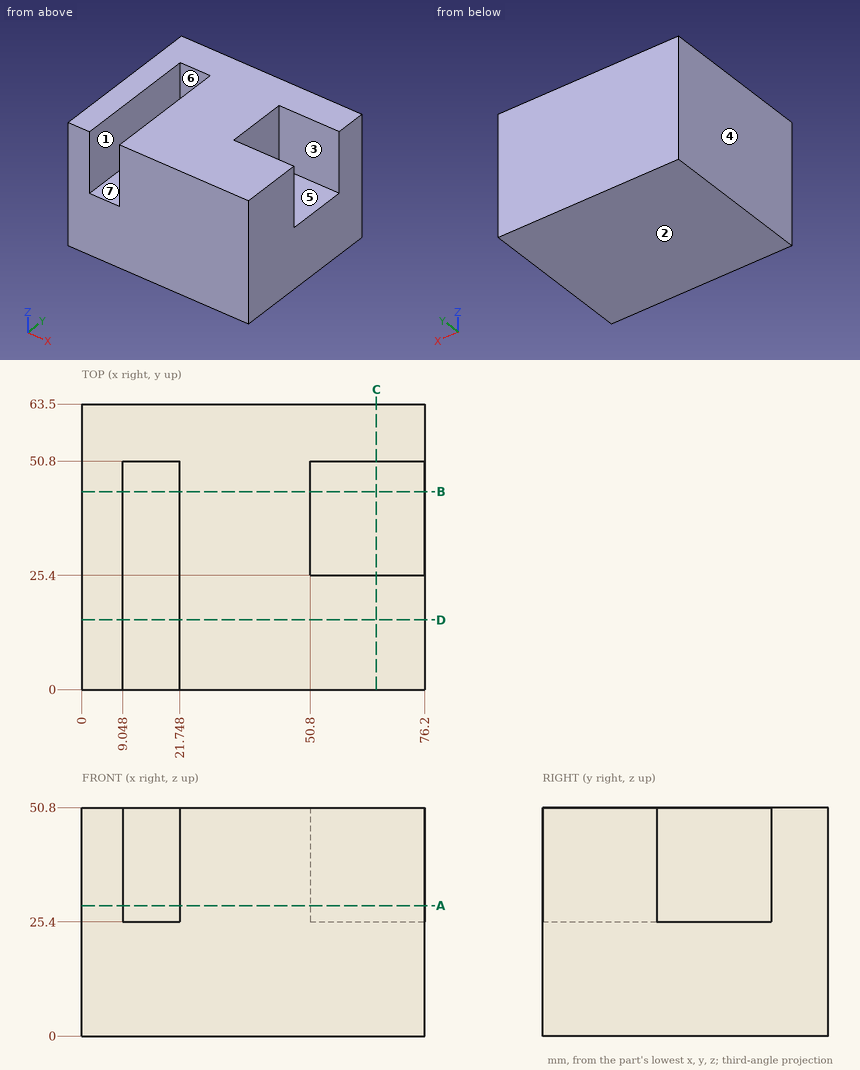
Geometry: see drawing. Coordinates: mm, zero at the bounding-box minimum. A direction names the side the tool comes from. Coordinates: 2 decimals unless noted, no trailing zeros. Order: outer loops, then holes, each group sorted by start corner. A loop starts at its lowest first (then second) coordinate and runs counter-clockwise, first axis right, second up. Notation, with made-up numbers: M 59.5,69.5 L 97.5,69.5 A17 ccw 97.5,84.5 Z; hole C -10.75,4.5 d3. An arc over 180 degrees is marked long. Answer in a Markdown table with one row per item. Add a question column.
Q1. Line query: L1, parallel to X at y = 44, z = 27; L2, parallel to X at y = 16, z = 49; L3, parallel to Y at x = 54.5, z = 43. Output: solid intervals per line, ascending.
Q2. Section query D-D on y = 15.5. Return the cut outline in (x, z), and give its area (3 significant figures).
Q3. Section query C-C on x = 65.5. Return the cut outline in (y, z).
Q4. Section query B-B on y = 44. Return the cut outline in (x, z).
Q5. Contact query for flat-ended pins moving along their axis: P1, Ø5, axis at x = 16, y = 11.5, coming from the +Z side; P2, Ø12, axis at y = 35, z = 44, coming from the +X side. Output: stop coordinate, or through.
Q6. Reachability of the marked faces 1, 2 and 3 from +Z, -Z, +X, -X, +Y, -Y: full face, straight path, thin tool, end or side. Return the list, or none.
Q7. Section query A-A on z = 29. Return the cut outline in (x, y).
Q8. Mould query, pull axis X, two halves, no side actions, for the marked faces 4, 5, 6 and 7. Classes: released by +X, released by -X, zero draft, split by the parting line, or undercut.
Completed:
| question | item | result |
|---|---|---|
| 1 | L1 | x = 0 to 9.05, 21.75 to 50.8 |
| 1 | L2 | x = 0 to 9.05, 21.75 to 76.2 |
| 1 | L3 | y = 0 to 25.4, 50.8 to 63.5 |
| 2 | outline | M 0,0 L 76.2,0 L 76.2,50.8 L 21.75,50.8 L 21.75,25.4 L 9.05,25.4 L 9.05,50.8 L 0,50.8 Z |
| 2 | area | 3,550 mm2 |
| 3 | outline | M 0,0 L 63.5,0 L 63.5,50.8 L 50.8,50.8 L 50.8,25.4 L 25.4,25.4 L 25.4,50.8 L 0,50.8 Z |
| 4 | outline | M 0,0 L 76.2,0 L 76.2,25.4 L 50.8,25.4 L 50.8,50.8 L 21.75,50.8 L 21.75,25.4 L 9.05,25.4 L 9.05,50.8 L 0,50.8 Z |
| 5 | P1 | stops at z = 25.4 |
| 5 | P2 | stops at x = 50.8 |
| 6 | face 1 | +Z, -Y |
| 6 | face 2 | -Z, +X, -X, +Y, -Y |
| 6 | face 3 | +Z, +X |
| 7 | outline | M 0,0 L 9.05,0 L 9.05,50.8 L 21.75,50.8 L 21.75,0 L 76.2,0 L 76.2,25.4 L 50.8,25.4 L 50.8,50.8 L 76.2,50.8 L 76.2,63.5 L 0,63.5 Z |
| 8 | face 4 | released by -X |
| 8 | face 5 | zero draft |
| 8 | face 6 | undercut |
| 8 | face 7 | undercut |
